The listing builds one solid part. Answer for the finished solid, in the listing's coordinates (mm). Round coordinates to 2 decimals unless told otherwise and drop trailing zeros. Write each loop counter-clockwise with the first axis right and the second up, starting at its lowest first coordinate (ties: lowest second). Pieces come first, ordered by that corner, then holes. Notation, with made-up numbers: (35.25, 1) - (89.25, 1) arc R14 ccw to (89.25, 15) - close; hole circle Ø4 at (86, -31.5). An arc over 180 degrees is marked (long way). Use a Markdown table: item, result. Add a question column.
1) Find the intervals of material crossed by probe 1 along Y at (x, z) = (-0.9, 90); probe 2 along Y at (x, z) = (-1.3, 106.68); probe 3 along Y at (x, z) = (-2.35, 39), in increasing order. Write a range as from..to.
2) Each of these flat-tipped pins is pushed along its axis until it touches: P1, Ø1.6, axis at x = -1.5, y = -145.5, coming from the +Z side; P2, Ø4.5, axis at y = 73.46, z = 169.8, coming from the +X side; P3, Ø1.7, axis at x = -1, y = -14.5, coming from the +Z side. Where does it stop, or does it pass through?
3) A cutting plane is placed at A-A (y = 35). Give the vertices of the cut face in (x, z) (3 decimals), then the cut area to 3 significant figures.
4) A cutting plane is placed at B-B (x = -0.85). State how many separate pieces and enclosed holes the cut face has, then the cut area to 3 significant figures.
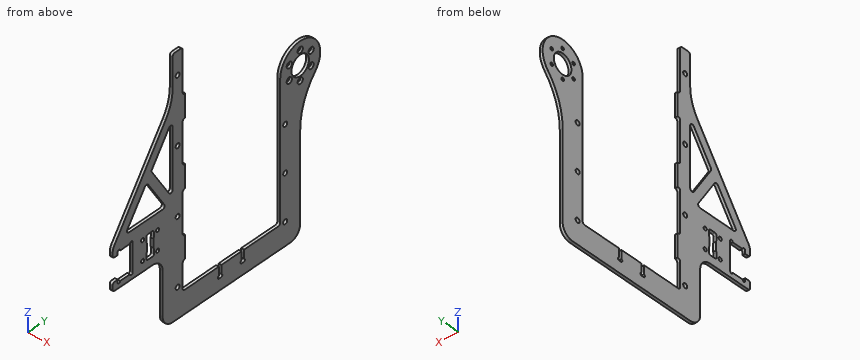
```python
from build123d import *

# Parameters (mm, degrees)
BASE_FLANGE1_DEPTH           = 3.175
SKETCH8_W                    = 12.7
SKETCH8_H                    = 3.302
CUT_EXTRUDE2_DEPTH           = 318.51984313
SKETCH11_R                   = 3.175
CUT_EXTRUDE4_DEPTH           = 318.51984313
SKETCH21_R                   = 2.5527
CUT_EXTRUDE5_DEPTH           = 318.51984313
SKETCH23_W                   = 25.4
SKETCH23_H                   = 3.175
TAB1_DEPTH                   = 3.175
CSK_FOR_M3_SFHCS1_AT_2_COUNT = 2
CSK_FOR_M3_SFHCS1_AT_2_PITCH = 16
CSK_FOR_M3_SFHCS1_AT_3_COUNT = 2
CSK_FOR_M3_SFHCS1_AT_3_PITCH = 27.712812921
CSK_FOR_M3_SFHCS1_AT_4_COUNT = 2
CSK_FOR_M3_SFHCS1_AT_4_PITCH = 32
CSK_FOR_M3_SFHCS1_AT_5_COUNT = 2
CSK_FOR_M3_SFHCS1_AT_5_PITCH = 27.712812921
CSK_FOR_M3_SFHCS1_AT_6_COUNT = 2
CSK_FOR_M3_SFHCS1_AT_6_PITCH = 16
SKETCH27_R                   = 2.0193
CUT_EXTRUDE6_DEPTH           = 318.51984313
CUT_EXTRUDE8_DEPTH           = 318.51984313
FILLET2_R                    = 12.7
SKETCH29_R                   = 11.1125
CUT_EXTRUDE9_DEPTH           = 318.51984313
BREAK_CORNER1_START          = -3.175
BREAK_CORNER1_DEPTH          = 3.175
FILLET1_R                    = 2.54
FILLET4_R                    = 50.8
CUT_EXTRUDE10_DEPTH          = 318.51984313
FILLET5_R                    = 2.54


# Read off the part's stored shape, not the designer's step: Break-Corner1
# Sheet-metal steps are written as plain solids
with BuildPart() as part:
    # Sketch1 → Base-Flange1 (new body)
    with BuildSketch(Plane(origin=(0, 0, 0), x_dir=(0, 0, -1), z_dir=(1, 0, 0))):
        with BuildLine():
            Line((0, -87.3125), (0, 87.3125))
            Line((0, 87.3125), (-110.597916699, 87.3125))
            ThreePointArc((-110.597916699, 87.3125), (-137.538685062, 92.233926782), (-160.999479175, 106.3625))
            ThreePointArc((-160.999479175, 106.3625), (-201.559524406, 96.292756121), (-177.8, 61.9125))
            Line((-177.8, 61.9125), (-25.4, 61.9125))
            Line((-25.4, 61.9125), (-25.4, -61.9125))
            Line((-25.4, -61.9125), (-279.4, -61.9125))
            Line((-279.4, -61.9125), (-279.4, -74.6125))
            Line((-279.4, -74.6125), (-228.6, -74.6125))
            Line((-228.6, -74.6125), (-118.11, -150.8125))
            Line((-118.11, -150.8125), (-108.585, -150.8125))
            Line((-108.585, -150.8125), (-108.585, -144.4625))
            Line((-108.585, -144.4625), (-111.76, -144.4625))
            Line((-111.76, -144.4625), (-111.76, -125.4125))
            Line((-111.76, -125.4125), (-80.01, -125.4125))
            Line((-80.01, -125.4125), (-80.01, -144.4625))
            Line((-80.01, -144.4625), (-83.185, -144.4625))
            Line((-83.185, -144.4625), (-83.185, -150.8125))
            Line((-83.185, -150.8125), (-73.66, -150.8125))
            Line((-73.66, -150.8125), (-73.66, -100.0125))
            ThreePointArc((-73.66, -100.0125), (-69.940256121, -91.032243879), (-60.96, -87.3125))
            Line((-60.96, -87.3125), (0, -87.3125))
        make_face()
    extrude(amount=-BASE_FLANGE1_DEPTH)

    # Sketch8 → Cut-Extrude2 (cut, through all)
    with BuildSketch(Plane(origin=(0, 0, 0), x_dir=(0, 0, -1), z_dir=(1, 0, 0))):
        with Locations((-19.05, 14.351)):
            Rectangle(SKETCH8_W, SKETCH8_H)
        with Locations((-19.05, -14.351)):
            Rectangle(SKETCH8_W, SKETCH8_H)
    extrude(amount=-CUT_EXTRUDE2_DEPTH, mode=Mode.SUBTRACT)

    # Sketch11 → Cut-Extrude4 (cut, through all)
    with BuildSketch(Plane(origin=(0, 0, 0), x_dir=(0, 0, -1), z_dir=(1, 0, 0))):
        with Locations((-177.8, 87.3125)):
            Circle(SKETCH11_R)
    extrude(amount=-CUT_EXTRUDE4_DEPTH, mode=Mode.SUBTRACT)

    # Sketch21 → Cut-Extrude5 (cut, through all)
    with BuildSketch(Plane(origin=(0, 0, 0), x_dir=(0, 0, -1), z_dir=(1, 0, 0))):
        with Locations((-33.02, -68.2625)):
            Circle(SKETCH21_R)
        with Locations((-106.68, -68.2625)):
            Circle(SKETCH21_R)
        with Locations((-180.34, -68.2625)):
            Circle(SKETCH21_R)
        with Locations((-254, -68.2625)):
            Circle(SKETCH21_R)
        with Locations((-25.4, 68.2625)):
            Circle(SKETCH21_R)
        with Locations((-76.2, 68.2625)):
            Circle(SKETCH21_R)
        with Locations((-127, 68.2625)):
            Circle(SKETCH21_R)
    extrude(amount=-CUT_EXTRUDE5_DEPTH, mode=Mode.SUBTRACT)

    # Sketch23 → Tab1 (add)
    with BuildSketch(Plane(origin=(0, 0, 0), x_dir=(0, 0, -1), z_dir=(1, 0, 0))):
        with Locations((-217.17, -60.325)):
            Rectangle(SKETCH23_W, SKETCH23_H)
        with Locations((-143.51, -60.325)):
            Rectangle(SKETCH23_W, SKETCH23_H)
        with Locations((-69.85, -60.325)):
            Rectangle(SKETCH23_W, SKETCH23_H)
    extrude(amount=-TAB1_DEPTH)

    # Sketch25 → CSK for M3 SFHCS1 (revolve, cut)
    with BuildSketch(Plane(origin=(0, 87.3125, 161.8), x_dir=(0, 0, -1), z_dir=(0, 1, 0))):
        Polygon((0, 0), (0, 3.175), (1.7, 3.175), (1.7, 1.66), (3.36, 0), align=None)
    csk_for_m3_sfhcs1 = revolve(axis=Axis((6.35, 87.3125, 161.8), (-1, 0, 0)), mode=Mode.SUBTRACT)

    # CSK for M3 SFHCS1 at 2: CSK for M3 SFHCS1 ×2
    with Locations(*[Vector(0, -0.8660254037844383, 0.5000000000000007) * (i * CSK_FOR_M3_SFHCS1_AT_2_PITCH) for i in range(1, CSK_FOR_M3_SFHCS1_AT_2_COUNT)]):
        add(csk_for_m3_sfhcs1, mode=Mode.SUBTRACT)

    # CSK for M3 SFHCS1 at 3: CSK for M3 SFHCS1 ×2
    with Locations(*[Vector(0, -0.5000000000000007, 0.8660254037844384) * (i * CSK_FOR_M3_SFHCS1_AT_3_PITCH) for i in range(1, CSK_FOR_M3_SFHCS1_AT_3_COUNT)]):
        add(csk_for_m3_sfhcs1, mode=Mode.SUBTRACT)

    # CSK for M3 SFHCS1 at 4: CSK for M3 SFHCS1 ×2
    with Locations(*[(0, 0, i * CSK_FOR_M3_SFHCS1_AT_4_PITCH) for i in range(1, CSK_FOR_M3_SFHCS1_AT_4_COUNT)]):
        add(csk_for_m3_sfhcs1, mode=Mode.SUBTRACT)

    # CSK for M3 SFHCS1 at 5: CSK for M3 SFHCS1 ×2
    with Locations(*[Vector(0, 0.500000000000001, 0.866025403784438) * (i * CSK_FOR_M3_SFHCS1_AT_5_PITCH) for i in range(1, CSK_FOR_M3_SFHCS1_AT_5_COUNT)]):
        add(csk_for_m3_sfhcs1, mode=Mode.SUBTRACT)

    # CSK for M3 SFHCS1 at 6: CSK for M3 SFHCS1 ×2
    with Locations(*[Vector(0, 0.8660254037844392, 0.49999999999999917) * (i * CSK_FOR_M3_SFHCS1_AT_6_PITCH) for i in range(1, CSK_FOR_M3_SFHCS1_AT_6_COUNT)]):
        add(csk_for_m3_sfhcs1, mode=Mode.SUBTRACT)

    # Sketch27 → Cut-Extrude6 (cut, through all)
    with BuildSketch(Plane(origin=(0, 0, 0), x_dir=(0, 0, -1), z_dir=(1, 0, 0))):
        with Locations((-85.09, -93.6625)):
            Circle(SKETCH27_R)
        with Locations(Location((-85.09, -112.7125, 0), (0, 0, 180))):
            Circle(SKETCH27_R)
        with Locations((-106.68, -112.7125)):
            Circle(SKETCH27_R)
        with Locations(Location((-106.68, -93.6625, 0), (0, 0, 180))):
            Circle(SKETCH27_R)
        with BuildLine():
            Line((-107.442, -98.45675), (-102.106618912, -98.45675))
            ThreePointArc((-102.106618912, -98.45675), (-101.283564844, -98.658721447), (-100.6475, -99.21875))
            Line((-100.6475, -99.21875), (-91.1225, -99.21875))
            ThreePointArc((-91.1225, -99.21875), (-90.486435156, -98.658721447), (-89.663381088, -98.45675))
            Line((-89.663381088, -98.45675), (-84.328, -98.45675))
            ThreePointArc((-84.328, -98.45675), (-83.070764143, -98.977514143), (-82.55, -100.23475))
            Line((-82.55, -100.23475), (-82.55, -106.14025))
            ThreePointArc((-82.55, -106.14025), (-83.070764143, -107.397485857), (-84.328, -107.91825))
            Line((-84.328, -107.91825), (-89.663381088, -107.91825))
            ThreePointArc((-89.663381088, -107.91825), (-90.486435156, -107.716278553), (-91.1225, -107.15625))
            Line((-91.1225, -107.15625), (-100.6475, -107.15625))
            ThreePointArc((-100.6475, -107.15625), (-101.283564844, -107.716278553), (-102.106618912, -107.91825))
            Line((-102.106618912, -107.91825), (-107.442, -107.91825))
            ThreePointArc((-107.442, -107.91825), (-108.699235857, -107.397485857), (-109.22, -106.14025))
            Line((-109.22, -106.14025), (-109.22, -100.23475))
            ThreePointArc((-109.22, -100.23475), (-108.699235857, -98.977514143), (-107.442, -98.45675))
        make_face()
    extrude(amount=-CUT_EXTRUDE6_DEPTH, mode=Mode.SUBTRACT)

    # Sketch28 → Cut-Extrude8 (cut, through all)
    with BuildSketch(Plane(origin=(0, 0, 0), x_dir=(0, 0, -1), z_dir=(1, 0, 0))):
        with BuildLine():
            Line((-111.76, -144.4625), (-111.76, -141.1605))
            ThreePointArc((-111.76, -141.1605), (-113.411, -142.8115), (-111.76, -144.4625))
        make_face()
        with BuildLine():
            Line((-80.01, -144.4625), (-80.01, -141.1605))
            ThreePointArc((-80.01, -141.1605), (-78.359, -142.8115), (-80.01, -144.4625))
        make_face()
        with BuildLine():
            Line((-80.01, -125.4125), (-80.01, -128.7145))
            ThreePointArc((-80.01, -128.7145), (-78.359, -127.0635), (-80.01, -125.4125))
        make_face()
        with BuildLine():
            Line((-111.76, -125.4125), (-111.76, -128.7145))
            ThreePointArc((-111.76, -128.7145), (-113.411, -127.0635), (-111.76, -125.4125))
        make_face()
        with BuildLine():
            ThreePointArc((-15.41705117, -14.351), (-14.290037971, -17.2085), (-13.163024773, -14.351))
            ThreePointArc((-13.163024773, -14.351), (-14.290037971, -11.4935), (-15.41705117, -14.351))
        make_face()
        with BuildLine():
            ThreePointArc((-15.41705117, 14.351), (-14.290037971, 11.4935), (-13.163024773, 14.351))
            ThreePointArc((-13.163024773, 14.351), (-14.290037971, 17.2085), (-15.41705117, 14.351))
        make_face()
    extrude(amount=-CUT_EXTRUDE8_DEPTH, mode=Mode.SUBTRACT)

    # Fillet2
    fillet2_edges = [part.edges().sort_by_distance(p)[0] for p in [
        (-1.5875, -87.3125, 0),
        (-1.5875, -150.8125, 118.11),
    ]]
    fillet(fillet2_edges, radius=FILLET2_R)

    # Sketch29 → Cut-Extrude9 (cut, through all)
    with BuildSketch(Plane.ZY.offset(3.175)):
        with Locations((177.8, 87.3125)):
            Circle(SKETCH29_R)
    extrude(amount=-CUT_EXTRUDE9_DEPTH, mode=Mode.SUBTRACT)

    # Break-Corner1 outline → Break-Corner1 (cut)
    with BuildSketch(Plane.YZ.offset(BREAK_CORNER1_START)):
        with BuildLine():
            ThreePointArc((87.3125, 12.7), (83.592756121, 3.719743879), (74.6125, 0))
            Line((74.6125, 0), (87.3125, 0))
            Line((87.3125, 0), (87.3125, 12.7))
        make_face()
    extrude(amount=BREAK_CORNER1_DEPTH, mode=Mode.SUBTRACT)

    # Fillet1
    fillet1_edges = [part.edges().sort_by_distance(p)[0] for p in [
        (-1.5875, -61.9125, 229.87),
        (-1.5875, -61.9125, 204.47),
        (-1.5875, -61.9125, 156.21),
        (-1.5875, -61.9125, 130.81),
        (-1.5875, -61.9125, 82.55),
        (-1.5875, -61.9125, 57.15),
        (-1.5875, -150.8125, 73.66),
        (-1.5875, -150.8125, 83.185),
        (-1.5875, -150.8125, 108.585),
        (-1.5875, -74.6125, 279.4),
        (-1.5875, -61.9125, 279.4),
        (-1.5875, -61.9125, 25.4),
        (-1.5875, 61.9125, 25.4),
    ]]
    fillet(fillet1_edges, radius=FILLET1_R)

    # Fillet4
    fillet4_edges = [part.edges().sort_by_distance(p)[0] for p in [
        (-1.5875, -74.6125, 228.6),
    ]]
    fillet(fillet4_edges, radius=FILLET4_R)

    # Sketch30 → Cut-Extrude10 (cut, through all)
    with BuildSketch(Plane.ZY.offset(3.175)):
        Polygon((124.46, -134.86266966), (163.882081016, -107.67502758), (124.46, -82.654490572), align=None)
        Polygon((211.822746006, -74.6125), (129.564117224, -74.6125), (172.400664991, -101.80014208), align=None)
    extrude(amount=-CUT_EXTRUDE10_DEPTH, mode=Mode.SUBTRACT)

    # Fillet5
    fillet5_edges = [part.edges().sort_by_distance(p)[0] for p in [
        (-1.5875, -74.6125, 211.822746006),
        (-1.5875, -101.80014208, 172.400664991),
        (-1.5875, -74.6125, 129.564117224),
        (-1.5875, -134.86266966, 124.46),
        (-1.5875, -82.654490572, 124.46),
        (-1.5875, -107.67502758, 163.882081016),
    ]]
    fillet(fillet5_edges, radius=FILLET5_R)


solid = part.part
```
Entries:
| question | item | result |
|---|---|---|
| 1 | probe 1 | y = -125.41..-107.89, -98.49..-61.91, 61.91..87.31 |
| 1 | probe 2 | y = -125.41..-114.73, -110.69..-107.92, -98.46..-95.68, -91.64..-70.82, -65.71..-61.91, 61.91..87.31 |
| 1 | probe 3 | y = -87.31..-61.91, 61.91..87.31 |
| 2 | P1 | stops at z = 126.97 |
| 2 | P2 | stops at x = -1.11 |
| 2 | P3 | stops at z = 12.7 |
| 3 | outline | (-3.175, 0) - (0, 0) - (0, 25.4) - (-3.175, 25.4) - close |
| 3 | area | 80.6 mm² |
| 4 | separate pieces | 1 |
| 4 | enclosed holes | 21 |
| 4 | area | 17,800 mm² |
